Autodesk Inventor part; units mm, degrees
ref_plane "YZ Plane" through (0, 0, 0) normal (1, 0, 0) x (0, 1, 0)
ref_plane "XZ Plane" through (0, 0, 0) normal (0, 1, 0) x (-1, 0, 0)
ref_plane "XY Plane" through (0, 0, 0) normal (0, 0, 1) x (1, 0, 0)
sketch "Sketch1" plane through (0, 0, 0) normal (0, 0, 1) x (1, 0, 0)
  line L0 (0, 0) -> (600, 0)
  line L1 (600, 0) -> (600, 250)
  line L2 (600, 250) -> (0, 250)
  line L3 (0, 250) -> (0, 0)
  dimension "d0" = 600
  dimension "d1" = 250
extrude "Extrusion1" add sketch "Sketch1" along normal blind 800
sketch "Sketch2" plane through (0, 0, 0) normal (0, -1, 0) x (1, 0, 0)
  line L0 (0, 0) -> (600, 0)
  line L1 (600, 0) -> (600, 800)
  line L2 (600, 800) -> (0, 800)
  line L3 (0, 800) -> (0, 0)
  line L4 (90, 710) -> (510, 710)
  line L5 (510, 710) -> (510, 90)
  line L6 (510, 90) -> (90, 90)
  line L7 (90, 90) -> (90, 710)
  line L8 (300, 710) -> (300, 90)
  line L9 (90, 400) -> (510, 400)
  line L10 (90, 710) -> (90, 400)
  line L11 (90, 400) -> (90, 90)
  line L12 (90, 555) -> (510, 555)
  line L13 (90, 245) -> (510, 245)
  line L14 (90, 710) -> (300, 710)
  line L15 (300, 710) -> (300, 555)
  line L16 (300, 555) -> (90, 555)
  line L17 (90, 555) -> (90, 710)
  line L18 (300, 555) -> (510, 555)
  line L19 (510, 555) -> (510, 710)
  line L20 (510, 710) -> (300, 710)
  line L21 (300, 710) -> (300, 555)
  line L22 (90, 555) -> (300, 555)
  line L23 (300, 555) -> (300, 400)
  line L24 (300, 400) -> (90, 400)
  line L25 (90, 400) -> (90, 555)
  line L26 (300, 400) -> (510, 400)
  line L27 (510, 400) -> (510, 555)
  line L28 (510, 555) -> (300, 555)
  line L29 (300, 555) -> (300, 400)
  line L30 (510, 400) -> (300, 400)
  line L31 (300, 400) -> (300, 245)
  line L32 (300, 245) -> (510, 245)
  line L33 (510, 245) -> (510, 400)
  line L34 (90, 400) -> (300, 400)
  line L35 (300, 400) -> (300, 245)
  line L36 (300, 245) -> (90, 245)
  line L37 (90, 245) -> (90, 400)
  line L38 (90, 90) -> (300, 90)
  line L39 (300, 90) -> (300, 245)
  line L40 (300, 245) -> (90, 245)
  line L41 (90, 245) -> (90, 90)
  line L42 (300, 245) -> (510, 245)
  line L43 (510, 245) -> (510, 90)
  line L44 (510, 90) -> (300, 90)
  line L45 (300, 90) -> (300, 245)
  line L46 (90, 632.5) -> (510, 632.5)
  line L47 (90, 477.5) -> (510, 477.5)
  line L48 (90, 322.5) -> (510, 322.5)
  line L49 (90, 167.5) -> (510, 167.5)
  line L50 (195, 710) -> (195, 90)
  line L51 (405, 710) -> (405, 90)
  circle A0 centre (195, 632.5) radius 20
  circle A1 centre (300, 632.5) radius 20
  circle A2 centre (405, 632.5) radius 20
  circle A3 centre (90, 632.5) radius 20
  circle A4 centre (510, 632.5) radius 20
  circle A5 centre (90, 477.5) radius 17.5
  circle A6 centre (195, 477.5) radius 17.5
  circle A7 centre (300, 477.5) radius 17.5
  circle A8 centre (405, 477.5) radius 17.5
  circle A9 centre (510, 477.5) radius 17.5
  circle A10 centre (195, 322.5) radius 20
  dimension "d4" = 90
  dimension "d5" = 40
  dimension "d6" = 40
  dimension "d7" = 40
  dimension "d8" = 40
  dimension "d9" = 40
  dimension "d10" = 35
  dimension "d11" = 35
  dimension "d12" = 35
  dimension "d13" = 35
  dimension "d14" = 35
  dimension "d15" = 40
extrude "Extrusion2" add sketch "Sketch2" along normal blind 15 contours A3 L46 L7 | L7 A3 | A0 L46 L50 | L50 L46 A0 | L46 A3 L7 | A1 L46 L8 | L8 L46 A1 | L50 A0 L46 | L46 A0 L50 | A2 L46 L51 | L51 L46 A2 | L46 A1 L8 | L8 A1 L46 | A4 L5 | L5 L46 A4 | L51 A2 L46 | L46 A2 L51 | L5 A4 L46
extrude "Extrusion3" add sketch "Sketch2" along normal blind 10 contours A5 L47 L7 | L7 A5 | L47 A5 L7 | A6 L47 L50 | L50 L47 A6 | L47 L50 A6 | A7 L47 L8 | L8 L47 A7 | L47 A6 L50 | L47 A7 L8 | L8 A7 L47 | A8 L47 L51 | L51 L47 A8 | L47 L51 A8 | A9 L5 | L5 L47 A9 | L47 A8 L51 | L5 A9 L47
extrude "Extrusion4" add sketch "Sketch2" along normal blind 20 contours A10 L50 L48 | L48 L50 A10 | A10 L48 L50 | L48 A10 L50
sketch "Sketch3" plane through (195, -10, 477.5) normal (0, -1, 0) x (1, 0, 0)
  circle A0 centre (-105, 0) radius 17.5
  circle A1 centre (-105, 0) radius 15
  circle A2 centre (0, 0) radius 17.5
  circle A3 centre (0, 0) radius 15
  circle A4 centre (105, 0) radius 17.5
  circle A5 centre (105, 0) radius 15
  circle A6 centre (210, 0) radius 17.5
  circle A7 centre (210, 0) radius 15
  circle A8 centre (315, 0) radius 17.5
  circle A9 centre (315, 0) radius 15
  point P0 (-195, -477.5)
  dimension "d22" = 30
  dimension "d23" = 30
  dimension "d24" = 30
  dimension "d25" = 30
  dimension "d26" = 30
extrude "Extrusion5" cut sketch "Sketch3" against normal blind 2 contours A1 | A3 | A5 | A7 | A9
sketch "Sketch4" plane through (195, -20, 322.5) normal (0, -1, 0) x (1, 0, 0)
  circle A0 centre (0, 0) radius 30
  point P0 (-195, -322.5)
  dimension "d29" = 60
extrude "Extrusion6" add sketch "Sketch4" along normal blind 30
properties part number "ControlPanel"
The model under review builds one solid part; all positions refer to its coordinate system, in mm. A direction names the side the tool comes from. Round coordinates to 2 decimals unless told otherwise and drop trailing zeros. Write each loop counter-clockwise with the first axis right and the second up, starting at its lowest first coordinate (ties: lowest second). Pieces come first, ordered by that corner, then holes. Notation, with made-up numbers: (88.5, -2) - (113.5, -2) arc R23 ccw to (113.5, 12) - close; hole circle Ø1 at (42.25, 1.5). An arc over 180 degrees is marked (long way). One line per question, with ' | ' between items.
Item 1: To check wall thickness, follow probe 1 along Z at (x, y) = (405, -8.35); probe 2 along Z at (x, y) = (195, -8.9); probe 3 along Y at (x, z) = (50, 36.5). State the ranges of each line that lie inside material, in increasing order.
Resolved:
probe 1: z = 460 to 462.5, 492.5 to 495, 612.5 to 652.5 | probe 2: z = 302.5 to 342.5, 460 to 462.5, 492.5 to 495, 612.5 to 652.5 | probe 3: y = 0 to 250
Item 2: Add section D-D, the plane x = 195. Give the boundary of the cut face in (y, z), then the cut area to 3 significant figures.
Resolved:
outline: (-50, 292.5) - (-20, 292.5) - (-20, 302.5) - (0, 302.5) - (0, 0) - (250, 0) - (250, 800) - (0, 800) - (0, 652.5) - (-15, 652.5) - (-15, 612.5) - (0, 612.5) - (0, 495) - (-10, 495) - (-10, 492.5) - (-8, 492.5) - (-8, 462.5) - (-10, 462.5) - (-10, 460) - (0, 460) - (0, 342.5) - (-20, 342.5) - (-20, 352.5) - (-50, 352.5) - close | area: 203,000 mm2
Item 3: Add section A-A, the plane x = 510. Give the boundary of the cut face in (y, z), then the cut area to 3 significant figures.
Resolved:
outline: (-15, 612.5) - (0, 612.5) - (0, 495) - (-10, 495) - (-10, 492.5) - (-8, 492.5) - (-8, 462.5) - (-10, 462.5) - (-10, 460) - (0, 460) - (0, 0) - (250, 0) - (250, 800) - (0, 800) - (0, 652.5) - (-15, 652.5) - close | area: 201,000 mm2
Item 4: For P1, Ø24, axis at x = 196.5, z = 472.5, coming from the -Y side; P2, Ø12, axis at x = 508, z = 625.5, coming from the -Y side; P3, Ø2, axis at y = 73, z = 424.5, coming from the -X side; P4, Ø8, axis at x = 349, z = 654.5, coming from the -Y side, all flat-tipped, find the tip position at first contact; note any pin that passes through.
Resolved:
P1: stops at y = -10 | P2: stops at y = -15 | P3: stops at x = 0 | P4: stops at y = 0
Item 5: The part is to be moulded in two halves that separate along X. For faces 1 (the face through (510, -8, 478)), 2 (the face through (190.664, -9.86, 342.024)), 3 (the face through (405, -15, 633)), say which applies: pulls with the +X half, pulls with the -X half, needs draft (parallel to the pull), parting line crosses it, or undercut.
Resolved:
face 1: undercut | face 2: parting line crosses it | face 3: needs draft
Item 6: Add section C-C, the plane z = 322.5. Give the boundary of the cut face in (x, y).
Resolved:
outline: (0, 0) - (175, 0) - (175, -20) - (165, -20) - (165, -50) - (225, -50) - (225, -20) - (215, -20) - (215, 0) - (600, 0) - (600, 250) - (0, 250) - close
Item 7: For faces 4 (the face through (296, 127, 800)), 5 (the face through (419.2, -10, 482.8)), 6 (the face through (405, -8, 478)), 7 (the face through (215, -20, 316)), list the 3-axis set-ups (+Z, -Z, +X, -X, +Y, -Y) from which the entire face can be reached by the end or side of a thin tool; tool diameter is ignored.
Resolved:
face 4: +Z, +X, -X, +Y, -Y | face 5: -Z, +X, -X, -Y | face 6: -Y | face 7: none
Item 8: Add section B-B, the plane z = 632.5. Give the boundary of the cut face in (x, y), then the cut area to 3 significant figures.
Resolved:
outline: (0, 0) - (70, 0) - (70, -15) - (110, -15) - (110, 0) - (175, 0) - (175, -15) - (215, -15) - (215, 0) - (280, 0) - (280, -15) - (320, -15) - (320, 0) - (385, 0) - (385, -15) - (425, -15) - (425, 0) - (490, 0) - (490, -15) - (530, -15) - (530, 0) - (600, 0) - (600, 250) - (0, 250) - close | area: 153,000 mm2
